from build123d import *

# Parameters (mm, degrees)
BOSS_EXTRUDE1_DEPTH = 190
SKETCH2_R           = 2.25
CUT_EXTRUDE1_DEPTH  = 3
SKETCH3_R           = 1.6
CUT_EXTRUDE2_DEPTH  = 3
SKETCH4_R           = 3.75
SKETCH4_R_2         = 1.5
CUT_EXTRUDE3_DEPTH  = 3
FILLET1_R           = 3


with BuildPart() as part:
    # Sketch1 → Boss-Extrude1 (new body)
    with BuildSketch(Plane(origin=(0, 0, 0), x_dir=(0, 0, -1), z_dir=(1, 0, 0))):
        Polygon((0, 0), (-20, 0), (-20, -3), (0, -3), (0, -35), (-20, -35), (-20, -38), (30, -38), (30, -35), (15, -35), align=None)
    extrude(amount=-BOSS_EXTRUDE1_DEPTH)

    # Sketch2 → Cut-Extrude1 (cut)
    with BuildSketch(Plane(origin=(0, 0, 0), x_dir=(1, 0, 0), z_dir=(0, 1, 0))):
        with Locations(Location((-185, -10, 0), (0, 0, 270))):
            Circle(SKETCH2_R)
        with Locations(Location((-125, -10, 0), (0, 0, 270))):
            Circle(SKETCH2_R)
        with Locations(Location((-65, -10, 0), (0, 0, 270))):
            Circle(SKETCH2_R)
        with Locations(Location((-5, -10, 0), (0, 0, 270))):
            Circle(SKETCH2_R)
    extrude(amount=-CUT_EXTRUDE1_DEPTH, mode=Mode.SUBTRACT)

    # Sketch3 → Cut-Extrude2 (cut)
    with BuildSketch(Plane.XZ.offset(38)):
        with Locations(Location((-116, 10, 0), (0, 0, 270))):
            Circle(SKETCH3_R)
        with Locations(Location((-74, 10, 0), (0, 0, 270))):
            Circle(SKETCH3_R)
        with Locations(Location((-182, 10, 0), (0, 0, 270))):
            Circle(SKETCH3_R)
        with Locations(Location((-170.5, 10, 0), (0, 0, 270))):
            Circle(SKETCH3_R)
        with Locations(Location((-19.5, 10, 0), (0, 0, 270))):
            Circle(SKETCH3_R)
        with Locations(Location((-8, 10, 0), (0, 0, 270))):
            Circle(SKETCH3_R)
    extrude(amount=-CUT_EXTRUDE2_DEPTH, mode=Mode.SUBTRACT)

    # Sketch4 → Cut-Extrude3 (cut)
    with BuildSketch(Plane(origin=(0, -35, 0), x_dir=(1, 0, 0), z_dir=(0, 1, 0))):
        with Locations(Location((-140, 21.5, 0), (0, 0, 270))):
            Circle(SKETCH4_R)
        with Locations(Location((-147.8, 21.5, 0), (0, 0, 270))):
            Circle(SKETCH4_R_2)
    extrude(amount=-CUT_EXTRUDE3_DEPTH, mode=Mode.SUBTRACT)

    # Fillet1
    fillet1_edges = [part.edges().sort_by_distance(p)[0] for p in [
        (-95, -35, 0),
        (-95, -3, 0),
        (-95, -35, -30),
        (-95, -35, 20),
        (-95, 0, 0),
    ]]
    fillet(fillet1_edges, radius=FILLET1_R - 0.0001)  # a hair under: the kernel refuses the full size


solid = part.part
For this review, take the finished solid that the model builds, in its own axes (mm). A direction names the side the tool comes from. Round coordinates to 2 decimals unless told otherwise and drop trailing zeros. Loops run counter-clockwise (first coordinate to the right, second up) from the corner with the lowest first, then second, coordinate; pieces in that order, holes last. Notation, with made-up numbers: (88.5, -25) - (117.5, -25) arc R13 cw to (117.5, -17) - close; hole circle Ø8 at (-8.5, 77). An arc over 180 degrees is marked (long way). Use one line per item in the form item = value.
1) We need section A-A on z = 14. Write out the cut boundary in (x, y), then the cut area to 3 significant figures.
Solutions:
outline = (-190, -38) - (0, -38) - (0, -35) - (-190, -35) - close; (-190, -3) - (0, -3) - (0, 0) - (-190, 0) - close
area = 1,140 mm2
2) We need section D-D on y = -21. Write out the cut boundary in (x, z).
Solutions:
outline = (-190, -9) - (0, -9) - (0, 0) - (-190, 0) - close
3) Tool access review of faces 4 (the face through (-67.196, -1.479, 9.512)), 5 (the face through (-94, -35, 10)), 6 (the face through (-17.914, -36.521, 10.208)), 7 (the face through (-94, 0, 11)): name each direction out of +Z, -Z, +X, -X, +Y, -Y from which nothing blocks a thin tool from reaching the whole face with its end or side.
Solutions:
face_4 = +Y
face_5 = +Z, +X, -X
face_6 = -Y
face_7 = +Z, -Z, +X, -X, +Y
4) Mouldability with a two-part tool opening along X and no side actions: class faces 1 (the face through (-190, -26, -3)), 2 (the face through (-94, -35, -21)), 3 (the face through (-127.196, -1.479, 9.512)) as pulls with the +X half, pulls with the -X half, needs draft (parallel to the pull), parting line crosses it, or undercut.
Solutions:
face_1 = pulls with the -X half
face_2 = needs draft
face_3 = undercut
5) Clearance check with flat-ended pins moving along their axes: P1, Ø10, axis at x = -140, z = -21.5, coming from the +Y side; P2, Ø7, axis at x = -185, z = 10, coming from the +Y side; P3, Ø1.9, axis at x = -74, z = 10, coming from the -Y side; P4, Ø6, axis at x = -77.5, y = -26, coming from the -Z side. State where each tip first meets the part, or that it passes through.
Solutions:
P1 = -35
P2 = 0
P3 = -3
P4 = -12.43
6) Wall thickness on probe 1 along X at (y, z) = (-1, 10); probe 2 along Y at (x, z) = (-44, 11); probe 3 along X at (y, z) = (-35.8, -21.5): over which ranges is each line inside the solid? List them lowest first.
Solutions:
probe_1 = -190 to -187.25, -182.75 to -127.25, -122.75 to -67.25, -62.75 to -7.25, -2.75 to 0
probe_2 = -38 to -35, -3 to 0
probe_3 = -190 to -149.3, -146.3 to -143.75, -136.25 to 0
